Autodesk Inventor part; units mm, degrees
ref_plane "YZ Plane" through (0, 0, 0) normal (1, 0, 0) x (0, 1, 0)
ref_plane "XZ Plane" through (0, 0, 0) normal (0, 1, 0) x (-1, 0, 0)
ref_plane "XY Plane" through (0, 0, 0) normal (0, 0, 1) x (1, 0, 0)
ref_plane "작업 평면1" through (0, 0, 0) normal (0, 0, 1) x (1, 0, 0)
sketch "스케치1" plane through (0, 0, 0) normal (0, 0, 1) x (1, 0, 0)
  arc A0 (20.1, 4.5766) -> (19.5808, 6.2636) centre (17.1, 4.5766) ccw
  line L0 (19.5808, 6.2636) -> (15.5953, 12.1246)
  arc A1 (15.5953, 12.1246) -> (13.9414, 13) centre (13.9414, 11) ccw
  line L1 (13, 13) -> (13.9414, 13)
  arc A2 (14.5, 11.5) -> (13, 13) centre (13, 11.5) ccw
  line L2 (14.5, -41.5) -> (14.5, 11.5)
  arc A3 (13.5, -42.5) -> (14.5, -41.5) centre (13.5, -41.5) ccw
  line L3 (-13.5, -42.5) -> (13.5, -42.5)
  arc A4 (-14.5, -41.5) -> (-13.5, -42.5) centre (-13.5, -41.5) ccw
  line L4 (-14.5, 11.5) -> (-14.5, -41.5)
  arc A5 (-13, 13) -> (-14.5, 11.5) centre (-13, 11.5) ccw
  line L5 (-13.9414, 13) -> (-13, 13)
  arc A6 (-13.9414, 13) -> (-15.5953, 12.1246) centre (-13.9414, 11) ccw
  line L6 (-15.5953, 12.1246) -> (-19.5808, 6.2636)
  arc A7 (-19.5808, 6.2636) -> (-20.1, 4.5766) centre (-17.1, 4.5766) ccw
  line L7 (-20.1, 4.5766) -> (-20.1, -39.6766)
  arc A8 (-20.1, -39.6766) -> (-19.5808, -41.3636) centre (-17.1, -39.6766) ccw
  line L8 (-19.5808, -41.3636) -> (-15.8929, -46.7869)
  arc A9 (-15.8929, -46.7869) -> (-13.4121, -48.1) centre (-13.4121, -45.1) ccw
  line L9 (-13.4121, -48.1) -> (13.4121, -48.1)
  arc A10 (13.4121, -48.1) -> (15.8929, -46.7869) centre (13.4121, -45.1) ccw
  line L10 (15.8929, -46.7869) -> (19.5808, -41.3636)
  arc A11 (19.5808, -41.3636) -> (20.1, -39.6766) centre (17.1, -39.6766) ccw
  line L11 (20.1, -39.6766) -> (20.1, 4.5766)
  circle A12 centre (-17.3, 4) radius 1.35
  circle A13 centre (-17.3, -18) radius 1.35
  circle A14 centre (-11, -45.3) radius 1.35
  circle A15 centre (17.3, 4) radius 1.35
  circle A16 centre (17.3, -18) radius 1.35
  circle A17 centre (11, -45.3) radius 1.35
  circle A18 centre (-17.3, -40) radius 1.35
  circle A19 centre (17.3, -40) radius 1.35
  arc A20 (-14.6, -41.5) -> (-13.5, -42.6) centre (-13.5, -41.5) ccw
  line L12 (-13.5, -42.6) -> (13.5, -42.6)
  arc A21 (13.5, -42.6) -> (14.6, -41.5) centre (13.5, -41.5) ccw
  line L13 (14.6, -41.5) -> (14.6, 11.5)
  arc A22 (14.6, 11.5) -> (12.2254, 12.9) centre (13, 11.5) ccw
  line L14 (12.2254, 12.9) -> (13.9414, 12.9)
  arc A23 (15.5126, 12.0684) -> (13.9414, 12.9) centre (13.9414, 11) ccw
  line L15 (15.5126, 12.0684) -> (19.4981, 6.2073)
  arc A24 (20, 4.5766) -> (19.4981, 6.2073) centre (17.1, 4.5766) ccw
  line L16 (20, 4.5766) -> (20, -39.6766)
  arc A25 (19.4981, -41.3073) -> (20, -39.6766) centre (17.1, -39.6766) ccw
  line L17 (19.4981, -41.3073) -> (15.8102, -46.7307)
  arc A26 (14.6, -47.7455) -> (15.8102, -46.7307) centre (13.4121, -45.1) ccw
  arc A27 (-15.8102, -46.7307) -> (-14.6, -47.7455) centre (-13.4121, -45.1) ccw
  line L18 (-15.8102, -46.7307) -> (-19.4981, -41.3073)
  arc A28 (-20, -39.6766) -> (-19.4981, -41.3073) centre (-17.1, -39.6766) ccw
  line L19 (-20, -39.6766) -> (-20, 4.5766)
  arc A29 (-19.4981, 6.2073) -> (-20, 4.5766) centre (-17.1, 4.5766) ccw
  line L20 (-19.4981, 6.2073) -> (-15.5126, 12.0684)
  arc A30 (-13.9414, 12.9) -> (-15.5126, 12.0684) centre (-13.9414, 11) ccw
  line L21 (-13.9414, 12.9) -> (-12.2254, 12.9)
  arc A31 (-12.2254, 12.9) -> (-14.6, 11.5) centre (-13, 11.5) ccw
  line L22 (-14.6, 11.5) -> (-14.6, -41.5)
  line L23 (-14.6, -42.6) -> (14.6, -42.6)
  line L24 (14.6, -42.6) -> (14.6, -48.1)
  line L25 (14.6, -48.1) -> (-14.6, -48.1)
  line L26 (-14.6, -48.1) -> (-14.6, -42.6)
  line L27 (-14.6, -48.1) -> (14.6, -48.1)
  line L28 (14.6, -48.1) -> (14.6, -57.1)
  line L29 (14.6, -57.1) -> (-14.6, -57.1)
  line L30 (-14.6, -57.1) -> (-14.6, -48.1)
  circle A32 centre (-11, -45.3) radius 1.4
  circle A33 centre (11, -45.3) radius 1.4
  line L31 (-6.05, -55.65) -> (6.05, -55.65)
  line L32 (6.05, -55.65) -> (6.05, -49.55)
  line L33 (6.05, -49.55) -> (-6.05, -49.55)
  line L34 (-6.05, -49.55) -> (-6.05, -55.65)
  line L35 (-6.05, -55.65) -> (6.05, -49.55) construction
  line L36 (6.05, -55.65) -> (-6.05, -49.55) construction
  line L37 (-14.6, -57.1) -> (14.6, -57.1)
  line L38 (14.6, -57.1) -> (14.6, -58.1)
  line L39 (14.6, -58.1) -> (-14.6, -58.1)
  line L40 (-14.6, -58.1) -> (-14.6, -57.1)
  circle A34 centre (9, -52.6) radius 1.35
  circle A35 centre (-9, -52.6) radius 1.35
  point P0 (0, 0)
  point P1 (0, -52.6)
  point P2 (-13.5, -42.6)
  dimension "d0" = 0.1
  dimension "d1" = 9
  dimension "d2" = 2.8
  dimension "d3" = 2.8
  dimension "d4" = 12.1
  dimension "d5" = 6.1
  dimension "d8" = 1
  dimension "d9" = 2.7
  dimension "d10" = 2.7
extrude "돌출2" add sketch "스케치1" along normal blind 6 contours L24 L25 A10 | A10 L9 A9 L26 L23 L12 L24 | L25 L28 L29 L30 L9 | L25 L26 A9 | L38 L39 L40 L29
sketch "스케치2" plane through (0, 0, 6) normal (0, 0, 1) x (1, 0, 0)
  line L0 (-6.05, -49.55) -> (6.05, -49.55)
  line L1 (6.05, -49.55) -> (6.05, -55.65)
  line L2 (-6.05, -55.65) -> (-6.05, -49.55)
  line L3 (6.05, -55.65) -> (-6.05, -55.65)
  circle A0 centre (6.05, -49.55) radius 1
  circle A1 centre (-6.05, -49.55) radius 1
  circle A2 centre (-6.05, -55.65) radius 1
  circle A3 centre (6.05, -55.65) radius 1
  point P0 (0, 0)
  point P1 (5.05, -55.65)
  point P2 (6.05, -54.65)
  dimension "d14" = 2
  dimension "d15" = 2
  dimension "d16" = 2
  dimension "d17" = 2
extrude "돌출3" cut sketch "스케치2" against normal blind 10 contours L2 A1 L0 | L0 A1 L2 | A0 L1 L0 | L0 L1 A0 | A2 L3 L2 | L2 L3 A2 | A3 L3 L1 picked at (5.393, -55.7298)
properties part number "chest connector_fixing part" material "PMMA 플라스틱"
The model under review builds one solid part; all positions refer to its coordinate system, in mm. A direction names the side the tool comes from. Give positions to 0.01 mm unless a question says otherwise; leave off trailing zeros. Write each loop counter-clockwise with the first axis right and the second up, starting at its lowest first coordinate (ties: lowest second). Pieces come first, ordered by that corner, then holes. Notation, with made-up numbers: (15.5, 77) -> (72.5, 77) arc R27 cw to (72.5, 100) -> close; hole circle Ø4 at (-30, 32.25). An arc over 180 degrees is marked (long way). Answer in a Markdown table with one row per item.
1) Add section B-B on y = -52.6. State the section outline as (x, z) points.
Worked answers:
| item | result |
|---|---|
| outline | (-14.6, 0) -> (-10.35, 0) -> (-10.35, 6) -> (-14.6, 6) -> close; (-7.65, 0) -> (-6.05, 0) -> (-6.05, 6) -> (-7.65, 6) -> close; (6.05, 0) -> (7.65, 0) -> (7.65, 6) -> (6.05, 6) -> close; (10.35, 0) -> (14.6, 0) -> (14.6, 6) -> (10.35, 6) -> close |
2) Add section A-A on x = 9. State the section outline as (y, z) points, plus the area to 3 significant figures.
Worked answers:
| item | result |
|---|---|
| outline | (-58.1, 0) -> (-53.95, 0) -> (-53.95, 6) -> (-58.1, 6) -> close; (-51.25, 0) -> (-42.6, 0) -> (-42.6, 6) -> (-51.25, 6) -> close |
| area | 76.8 mm² |
3) Tool access review of faces 4 (the flat face through (6.05, -53, 3)), 5 (the flat face through (0, -42.6, 3)): name each direction out of +Z, -Z, +X, -X, +Y, -Y from which nothing blocks a thin tool from reaching the whole face with its end or side.
Worked answers:
| item | result |
|---|---|
| face 4 | +Z, -Z |
| face 5 | +Z, -Z, +X, -X, +Y |
4) For L1, parallel to X at y = -52.5, z = 0.45; L2, parallel to X at y = -49.5, z = 5.15; L3, parallel to Y at x = -11, z = 2.25, list the stretches that pass through material, from the lowest coordinate up. Write a range as [from, to].
Worked answers:
| item | result |
|---|---|
| L1 | [-14.6, -10.35], [-7.65, -6.05], [6.05, 7.65], [10.35, 14.6] |
| L2 | [-14.6, -7.05], [-5.05, 5.05], [7.05, 14.6] |
| L3 | [-58.1, -46.7], [-43.9, -42.6] |
5) Add section D-D on y = -45.3. State the section outline as (x, z) points.
Worked answers:
| item | result |
|---|---|
| outline | (-14.6, 0) -> (-12.4, 0) -> (-12.4, 6) -> (-14.6, 6) -> close; (-9.6, 0) -> (9.6, 0) -> (9.6, 6) -> (-9.6, 6) -> close; (12.4, 0) -> (14.6, 0) -> (14.6, 6) -> (12.4, 6) -> close |
6) Mouldability with a two-part tool opening along Y and no side actions: class faces 1 (the flat face through (0, -58.1, 3)), 2 (the cylindrical face through (6.733, -56.38, 3.042)), 3 (the flat face through (0, -49, 0)) as +Y half, -Y half, draft (parallel to the pull), parting line (faces both ways), or undercut.
Worked answers:
| item | result |
|---|---|
| face 1 | -Y half |
| face 2 | undercut |
| face 3 | draft |
7) Add section C-C on z = 2.25. State the section outline as (x, y) points, plus the area to 3 significant figures.
Worked answers:
| item | result |
|---|---|
| outline | (-14.6, -58.1) -> (14.6, -58.1) -> (14.6, -42.6) -> (-14.6, -42.6) -> close; hole circle Ø2.8 at (-11, -45.3); hole circle Ø2.7 at (-9, -52.6); hole (-6.05, -54.65) arc R1 ccw (long way) to (-5.05, -55.65) -> (5.05, -55.65) arc R1 ccw (long way) to (6.05, -54.65) -> (6.05, -50.55) arc R1 ccw (long way) to (5.05, -49.55) -> (-5.05, -49.55) arc R1 ccw (long way) to (-6.05, -50.55) -> close; hole circle Ø2.7 at (9, -52.6); hole circle Ø2.8 at (11, -45.3) |
| area | 346 mm² |
8) Clearance check with a flat-ended pin moving along its axis: P1, Ø2, axis at x = -11, y = -45.3, coming from the -Z side. State where the tip first meets the part, or that it passes through.
Worked answers:
| item | result |
|---|---|
| P1 | through |
